from build123d import *

# Parameters (mm, degrees)
F0_W     = 6.7567604338
F0_H     = 5
F3_DEPTH = 5
F6_DEPTH = 25
F7_DEPTH = 25


# Not quite as in the source:
# - a feature names something its author has since deleted; it is built from what else it names


with BuildPart() as f1:
    # F0 (on Front) → F1 (revolve)
    with BuildSketch(Plane.XZ):
        with Locations((9.3783802169, 15)):
            Rectangle(F0_W, F0_H)
    revolve(axis=Axis((0, 0, -3.2319817692), (0, 0, -1)))

    # F2 (on face) → F3 (cut, through all)
    with BuildSketch(Plane.XY.offset(17.5)):
        with BuildLine():
            ThreePointArc((1, 12.7175051313), (0, 12.7567604338), (-1, 12.7175051313))
            Line((-1, 12.7175051313), (-1, 5.9160797831))
            ThreePointArc((-1, 5.9160797831), (0, 6), (1, 5.9160797831))
            Line((1, 5.9160797831), (1, 12.7175051313))
        make_face()
        with BuildLine():
            Line((-4.623475383, 3.8240652953), (-10.5136825165, 7.2247779694))
            ThreePointArc((-10.5136825165, 7.2247779694), (-11.0476786056, 6.3783802169), (-11.5136825165, 5.4927271619))
            Line((-11.5136825165, 5.4927271619), (-5.623475383, 2.0920144878))
            ThreePointArc((-5.623475383, 2.0920144878), (-5.1961524227, 3), (-4.623475383, 3.8240652953))
        make_face()
        with BuildLine():
            Line((-5.623475383, -2.0920144878), (-11.5136825165, -5.4927271619))
            ThreePointArc((-11.5136825165, -5.4927271619), (-11.0476786056, -6.3783802169), (-10.5136825165, -7.2247779694))
            Line((-10.5136825165, -7.2247779694), (-4.623475383, -3.8240652953))
            ThreePointArc((-4.623475383, -3.8240652953), (-5.1961524227, -3), (-5.623475383, -2.0920144878))
        make_face()
        with BuildLine():
            Line((-1, -5.9160797831), (-1, -12.7175051313))
            ThreePointArc((-1, -12.7175051313), (0, -12.7567604338), (1, -12.7175051313))
            Line((1, -12.7175051313), (1, -5.9160797831))
            ThreePointArc((1, -5.9160797831), (0, -6), (-1, -5.9160797831))
        make_face()
        with BuildLine():
            ThreePointArc((10.5136825165, -7.2247779694), (11.0476786056, -6.3783802169), (11.5136825165, -5.4927271619))
            Line((11.5136825165, -5.4927271619), (5.623475383, -2.0920144878))
            ThreePointArc((5.623475383, -2.0920144878), (5.1961524227, -3), (4.623475383, -3.8240652953))
            Line((4.623475383, -3.8240652953), (10.5136825165, -7.2247779694))
        make_face()
        with BuildLine():
            ThreePointArc((11.5136825165, 5.4927271619), (11.0476786056, 6.3783802169), (10.5136825165, 7.2247779694))
            Line((10.5136825165, 7.2247779694), (4.623475383, 3.8240652953))
            ThreePointArc((4.623475383, 3.8240652953), (5.1961524227, 3), (5.623475383, 2.0920144878))
            Line((5.623475383, 2.0920144878), (11.5136825165, 5.4927271619))
        make_face()
    extrude(amount=-F3_DEPTH, mode=Mode.SUBTRACT)


with BuildPart() as f4:
    # F0 (on Front) → F4 (revolve)
    with BuildSketch(Plane.XZ):
        Polygon((6, 30), (6, 17.5), (12.7567604338, 17.5), (11, 30), align=None)
    revolve(axis=Axis((0, 0, -3.2319817692), (0, 0, -1)))


with BuildPart() as f4b:
    # F0 (on Front) → F4, piece 2 (revolve)
    with BuildSketch(Plane.XZ):
        Polygon((6, 12.5), (6, 0), (11, 0), (12.7567604338, 12.5), align=None)
    revolve(axis=Axis((0, 0, -3.2319817692), (0, 0, -1)))


with BuildPart() as f1_1:
    add(f1.part)

    # F5: union F4b, F4
    add(f4b.part)
    add(f4.part)

    # F6 (cut): faces of the model
    f6_faces = [f1_1.faces().sort_by_distance(p)[0] for p in [
        (0, -9.3578583369, 17.5),
        (8.1041430447, 4.6789291684, 17.5),
        (-8.1041430447, 4.6789291684, 17.5),
    ]]
    extrude(f6_faces, amount=-F6_DEPTH, mode=Mode.SUBTRACT)

    # F7 (cut): faces of the model
    f7_faces = [f1_1.faces().sort_by_distance(p)[0] for p in [
        (8.1041430447, -4.6789291684, 12.5),
        (0, 9.3578583369, 12.5),
        (-8.1041430447, -4.6789291684, 12.5),
    ]]
    extrude(f7_faces, amount=-F7_DEPTH, mode=Mode.SUBTRACT)


solid = f1_1.part
Here's how the part is built. I have some questions about the finished solid (model axes, mm). A direction names the side the tool comes from. Coordinates: 2 decimals unless noted, no trailing zeros. Write each loop counter-clockwise with the first axis right and the second up, starting at its lowest first coordinate (ties: lowest second). Pieces come first, ordered by that corner, then holes.
Item 1: If I drill on line 1 (X direction, y = -4.25, z = 7.5); line 2 (X direction, y = -2.5, z = 22.5); line 3 (X direction, y = 0, z = 7.25), over which ranges is the centre line in solid material (lowest first)?
Item 2: On a 3-axis mill with a long thin cutter (end or side, diameter ignored), from which of +Z, -Z, +X, -X, +Y, -Y can I reach the whole of each face in a straight line? I mean faces 1 (the flat face through (1, 9, 9)), 2 (the flat face through (-7.61, -5.55, 8.87)), 3 (the flat face through (-7, 3, 0)), 4 (the flat face through (8, 5, 12.5)), 5 (the cylindrical face through (6.447, -11.008, 15.035)). Say none if no direction works.
Item 3: I want a section at D-D on z = 7.5. Write out the boundary of the cut face in (x, y).
Item 4: I want a section at B-B on z = 16.5. Write out the boundary of the cut face in (x, y), and give its area (3 significant figures).
Item 5: I want a section at A-A on x = 0. Write out the boundary of the cut face in (y, z).
Item 6: If we mould it in two halves opening along X, with no side actions, what happens to faces 6 (the flat face through (8.61, -3.816, 8.872)), 7 (the cylindrical face through (-12.757, -0.079, 15.035)), 8 (the conical face through (0.16, -11.89, 6.34)), 9 (the flat face through (8.53, 3.77, 21.13))? For each: +X half, -X half, draft (parallel to the pull), parting line (faces both ways), or undercut.
Item 7: Will these pins go through, and if not, where does the flat tip stop? pin 1 (10 mm diameter, centred on y = -9.5, z = 24, fed in from +X); pin 2 (7.5 mm diameter, centred on y = -10, z = 19.5, fed in from -X); pin 3 (2 mm diameter, centred on y = -10.5, z = 25, fed in from +X); pin 4 (11 mm diameter, centred on x = 0, y = 0, fed in from +Z).
Item 8: I want a section at C-C on z = 26. Write out the boundary of the cut face in (x, y).
Findings below:
1. line 1: x = -11.28 to -9.36, -5.36 to -4.24, 4.24 to 5.36, 9.36 to 11.28
1. line 2: x = -11.79 to -5.45, 5.45 to 11.79
1. line 3: x = -12.02 to -6, 6 to 12.02
2. face 1: -Z, +Y
2. face 2: -Z
2. face 3: -Z, +X, -X, +Y, -Y
2. face 4: +Z
2. face 5: +Z, -Z, +X, -Y
3. outline: (-10.9, -5.14) - (-5.62, -2.09) arc R6 cw to (-1, 5.92) - (-1, 12.01) arc R12.05 ccw to start; (-9.9, -6.87) arc R12.05 ccw to (9.9, -6.87) - (4.62, -3.82) arc R6 cw to (-4.62, -3.82) - close; (1, 5.92) arc R6 cw to (5.62, -2.09) - (10.9, -5.14) arc R12.05 ccw to (1, 12.01) - close
4. outline: (-11.51, -5.49) - (-5.62, -2.09) arc R6 cw to (-5.62, 2.09) - (-11.51, 5.49) arc R12.76 ccw to start; (-10.51, -7.22) arc R12.76 ccw to (-1, -12.72) - (-1, -5.92) arc R6 cw to (-4.62, -3.82) - close; (-10.51, 7.22) - (-4.62, 3.82) arc R6 cw to (-1, 5.92) - (-1, 12.72) arc R12.76 ccw to start; (1, -12.72) arc R12.76 ccw to (10.51, -7.22) - (4.62, -3.82) arc R6 cw to (1, -5.92) - close; (1, 5.92) arc R6 cw to (4.62, 3.82) - (10.51, 7.22) arc R12.76 ccw to (1, 12.72) - close; (5.62, -2.09) - (11.51, -5.49) arc R12.76 ccw to (11.51, 5.49) - (5.62, 2.09) arc R6 cw to start
4. area: 317 mm2
5. outline: (-12.76, 12.5) - (-11, 0) - (-6, 0) - (-6, 12.5) - close; (6, 17.5) - (12.76, 17.5) - (11, 30) - (6, 30) - close
6. face 6: undercut
6. face 7: -X half
6. face 8: parting line
6. face 9: undercut
7. pin 1: stops at x = 11.09
7. pin 2: stops at x = -10.88
7. pin 3: stops at x = 6.85
7. pin 4: passes through
8. outline: (-10.48, 4.89) arc R11.56 ccw to (-1, -11.52) - (-1, -5.92) arc R6 cw to (-5.62, 2.09) - close; (-9.48, 6.63) - (-4.62, 3.82) arc R6 cw to (4.62, 3.82) - (9.48, 6.63) arc R11.56 ccw to start; (1, -11.52) arc R11.56 ccw to (10.48, 4.89) - (5.62, 2.09) arc R6 cw to (1, -5.92) - close
